```python
from build123d import *

# Parameters (mm, degrees)
F1_DEPTH = 30.988
F2_W     = 12.6881152391
F2_H     = 10.5545610582
F3_DEPTH = 25.4
F4_DEPTH = 25.4
F5_R     = 4.1061921306
F6_DEPTH = 25.4
F7_R     = 14.1038356314


with BuildPart() as f1:
    # F0 (on Front) → F1 (new body)
    with BuildSketch(Plane.XZ):
        Polygon((11.8142822757, 0), (0, 0), (0, -25.6347749382), (76.0126635432, -25.6347749382), (76.0126635432, -14.9350436404), (11.8142822757, -14.9350436404), align=None)
    extrude(amount=F1_DEPTH)

    # F2 (on face) → F3 (cut)
    with BuildSketch(Plane.XY.offset(-14.9350436404)):
        with Locations((45.7378029823, -25.7107194709)):
            Rectangle(F2_W, F2_H)
    extrude(amount=-F3_DEPTH, mode=Mode.SUBTRACT)

    # F2 (on face) → F4 (cut)
    with BuildSketch(Plane.XY.offset(-14.9350436404)):
        Polygon((76.0126635432, 0), (65.1537999511, 0), (76.0126635432, -9.4870273024), align=None)
        with Locations((45.7378029823, -25.7107194709)):
            Rectangle(F2_W, F2_H)
    extrude(amount=-F4_DEPTH, mode=Mode.SUBTRACT)

    # F5 (on face) → F6 (cut)
    with BuildSketch(Plane.YZ.offset(11.8142822757)):
        with Locations((-16.0313341767, -7.6476014219)):
            Circle(F5_R)
    extrude(amount=-F6_DEPTH, mode=Mode.SUBTRACT)

    # F7
    f7_edges = [f1.edges().sort_by_distance(p)[0] for p in [
        (5.907141, -30.988, 0),
        (5.907141, 0, 0),
    ]]
    fillet(f7_edges, radius=F7_R)


solid = f1.part
```
CAD build for the part. Positions are in the model's coordinates, mm. A direction names the side the tool comes from. Coordinates: 2 decimals unless noted, no trailing zeros. Order: outer loops, then holes, each group sorted by start corner. A loop starts at its lowest first (then second) coordinate and runs counter-clockwise, first axis right, second up. Notation, with made-up numbers: M 34,55.25 L 87,55.25 A16 ccw 87,65.25 Z; hole C 45,12 d9. An arc over 180 degrees is marked long. Write each question's results on one line, items separated by ' | '. Start each with the question number.
Q1. Cut at D-D (y = -18.5). List the corners of the cut face in (x, z), then the cut area to 3 significant figures.
Q2. Drill centre lines: probe 1 along X at (y, z) = (-24, -22); probe 2 along Z at (x, y) = (11.5, -16); probe 3 along Z at (x, y) = (41, -2). Where is each one in solid material? Low to high. Write a range as from..to.
Q3. Pull direction X, two halves, no side cores. Call faces 1 (the flat face through (19, -30.988, -20)), 2 (the flat face through (52.082, -26, -20)), 3 (the flat face through (76.013, -20, -20)), 4 (the flat face through (39.394, -26, -20)): +X half, -X half, draft (parallel to the pull), parting line (faces both ways), or undercut.
Q4. Cut at C-C (x = 51). List the corners of the cut face in (y, z).
Q5. Cut at A-A (y = -27.5). List the corners of the cut face in (x, z), then the cut area to 3 significant figures.
Q6. Cut at B-B (z = -19). List the corners of the cut face in (x, y), then the cut area to 3 significant figures.
Q7. Flat gauge pins, fed straight in: P1, Ø12, axis at x = 45.5, z = -18.5, coming from the -Y side; P2, Ø6, axis at x = 27.5, y = -24.5, coming from the +Z side; P3, Ø8, axis at y = -27, z = -3.5, coming from the +X side. Where does each tip first touch, or does it go through?
Q8. Which spindle directions (+Z, -Z, +X, -X, +Y, -Y) get a long thin tool onto all of the face, cutting with end or side? Do faces 5 (the flat face through (11.814, -11.8, -9.2)), 6 (the flat face through (70.51, -4.68, -20.21)), 7 (the flat face through (46, -20.433, -20)). Say none if no direction does.
Found:
1) outline: M 0,-25.63 L 76.01,-25.63 L 76.01,-14.94 L 11.81,-14.94 L 11.81,-10.93 L 0,-10.93 Z; M 0,-4.37 L 11.81,-4.37 L 11.81,-0.09 L 0,-0.09 Z | area: 911 mm²
2) probe 1: 0..39.39, 52.08..76.01 | probe 2: -25.63..-11.75, -3.54..0 | probe 3: -25.63..-14.94
3) face 1: draft | face 2: undercut | face 3: +X half | face 4: undercut
4) outline: M -20.43,-25.63 L 0,-25.63 L 0,-14.94 L -20.43,-14.94 Z
5) outline: M 0,-25.63 L 39.39,-25.63 L 39.39,-14.94 L 11.81,-14.94 L 11.81,-4.82 L 0,-4.82 Z; M 52.08,-25.63 L 76.01,-25.63 L 76.01,-14.94 L 52.08,-14.94 Z | area: 797 mm²
6) outline: M 0,-30.99 L 39.39,-30.99 L 39.39,-20.43 L 52.08,-20.43 L 52.08,-30.99 L 76.01,-30.99 L 76.01,-9.49 L 65.15,0 L 0,0 Z | area: 2,170 mm²
7) P1: y = -20.43 | P2: z = -14.94 | P3: x = 11.81
8) face 5: +Z, +X, +Y, -Y | face 6: +Z, -Z, +X, +Y | face 7: +Z, -Z, -Y
